```python
from build123d import *

# Parameters (mm, degrees)
SURFACE_EXTRUDE1_1_DEPTH = 140
THICKEN1_T2              = 2
SKETCH2_R                = 2
CUT_EXTRUDE2_DEPTH       = 142.774468788


with BuildPart() as body_1:
    # Surface-Extrude1: a surface, the sketch's curves swept straight by 140 mm
    with BuildLine(Plane(origin=(0, 0, 0), x_dir=(0, 0, -1), z_dir=(1, 0, 0)), mode=Mode.PRIVATE) as surface_extrude1_1_path:
        Line((0, 10), (0, 0))
        Line((0, 0), (20, 0))
    surface_extrude1_1 = Shell.extrude(surface_extrude1_1_path.wire(), (1 * SURFACE_EXTRUDE1_1_DEPTH, 0 * SURFACE_EXTRUDE1_1_DEPTH, 0 * SURFACE_EXTRUDE1_1_DEPTH))
    add(Solid.thicken(surface_extrude1_1, -THICKEN1_T2))

    # Sketch2 → Cut-Extrude2 (cut, through all)
    with BuildSketch(Plane(origin=(0, 0, 0), x_dir=(-1, 0, 0), z_dir=(0, 0, -1))):
        with Locations((-130, 5)):
            Circle(SKETCH2_R)
        with Locations(Location((-10, 5, 0), (0, 0, 180))):
            Circle(SKETCH2_R)
    extrude(amount=-CUT_EXTRUDE2_DEPTH, mode=Mode.SUBTRACT)


solid = body_1.part
```
Source: CAD feature listing. Evaluate the final solid. Frame: model axes, mm. A direction names the side the tool comes from. Round coordinates to 2 decimals unless told otherwise and drop trailing zeros. Write each loop counter-clockwise with the first axis right and the second up, starting at its lowest first coordinate (ties: lowest second). Pieces come first, ordered by that corner, then holes. Notation, with made-up numbers: M 34,71 L 87,71 A15 cw 87,88 Z; hole C 44.25,-24 d4. An arc over 180 degrees is marked long. Answer as a JSON object with one key per item and string values. Group by question number.
(1) Section query A-A on y = 5. Output: boundary loops of the cut face in (x, z), then the cut area to 3 significant figures.
(2) Reachability of faces 5 (the flat face through (69, 0, -10)), 6 (the flat face through (69, -2, -9)) from +Z, -Z, +X, -X, +Y, -Y: full face, straight path, thin tool, end or side. Return the list, or none.
(3) Ray query, line 1 (Y direction, x = 130, z = 0.9); line 2 (Y direction, x = 105, z = -9.5); line 3 (X direction, y = 4.5, z = 0.5). Return the intervals inside material, ascending. Write a range as [from, to].
(4) Section query B-B on x = 130. Output: boundary loops of the cut face in (y, z).
(5) Mould query, pull axis X, two halves, no side actions, for faces 1 (the cylindrical face through (8.4, 6.2, 1)), 2 (the flat face through (69, 4, 2)), 3 (the flat face through (140, -0.5, -5.7)), 4 (the cylindrical face through (132, 5, 1)). Classes: +X half, -X half, draft (parallel to the pull), parting line (faces both ways), or undercut.
(6) Section query D-D on z = -6. Output: boundary loops of the cut face in (x, y), then the cut area to 3 significant figures.
(7) Section query C-C on x = 21. Output: boundary loops of the cut face in (y, z), then the cut area to 3 significant figures.
(8) First-contact query: pin 1 (1.5 mm diameter, centred on x = 104, y = 5.5, fed in from -Z); pin 2 (8 mm diameter, centred on x = 50.5, z = -13, fed in from +Y); pin 3 (3 mm diameter, centred on y = 1, z = -2.5, fed in from -X). Flat tips, straight axial feed; report the tip coordinate or a pass-through.
Computed values:
{
 "1": {"outline": "M 0,0 L 8,0 L 8,2 L 0,2 Z; M 12,0 L 128,0 L 128,2 L 12,2 Z; M 132,0 L 140,0 L 140,2 L 132,2 Z", "area": "264 mm^2"},
 "2": {"face 5": "-Z, +X, -X, +Y", "face 6": "+Z, -Z, +X, -X, -Y"},
 "3": {"line 1": "[-2, 3], [7, 10]", "line 2": "[-2, 0]", "line 3": "[0, 8.06], [11.94, 128.06], [131.94, 140]"},
 "4": {"outline": "M -2,-20 L 0,-20 L 0,0 L 3,0 L 3,2 L -2,2 Z; M 7,0 L 10,0 L 10,2 L 7,2 Z"},
 "5": {"face 1": "undercut", "face 2": "draft", "face 3": "+X half", "face 4": "undercut"},
 "6": {"outline": "M 0,-2 L 140,-2 L 140,0 L 0,0 Z", "area": "280 mm^2"},
 "7": {"outline": "M -2,-20 L 0,-20 L 0,0 L 10,0 L 10,2 L -2,2 Z", "area": "64.0 mm^2"},
 "8": {"pin 1": "z = 0", "pin 2": "y = 0", "pin 3": "x = 0"}
}
